Print and shaded views of the part. All mm, measured from the part's lowest x, y and z. A direction names the side the tool comes from. Round coordinates to 2 decimals unless told otherwise and drop trailing zeros. Loops run counter-clockwise (first coordinate to the right, second up) from the corner with the lowest first, then second, coordinate; pieces in that order, holes last. Notation, with made-up numbers: (22.25, 38.5) -> (56.25, 38.5) arc R28 ccw to (56.25, 71.5) -> close; hole circle Ø2 at (-31, -4). An arc over 180 degrees is marked (long way). Use a Markdown table: item, result.
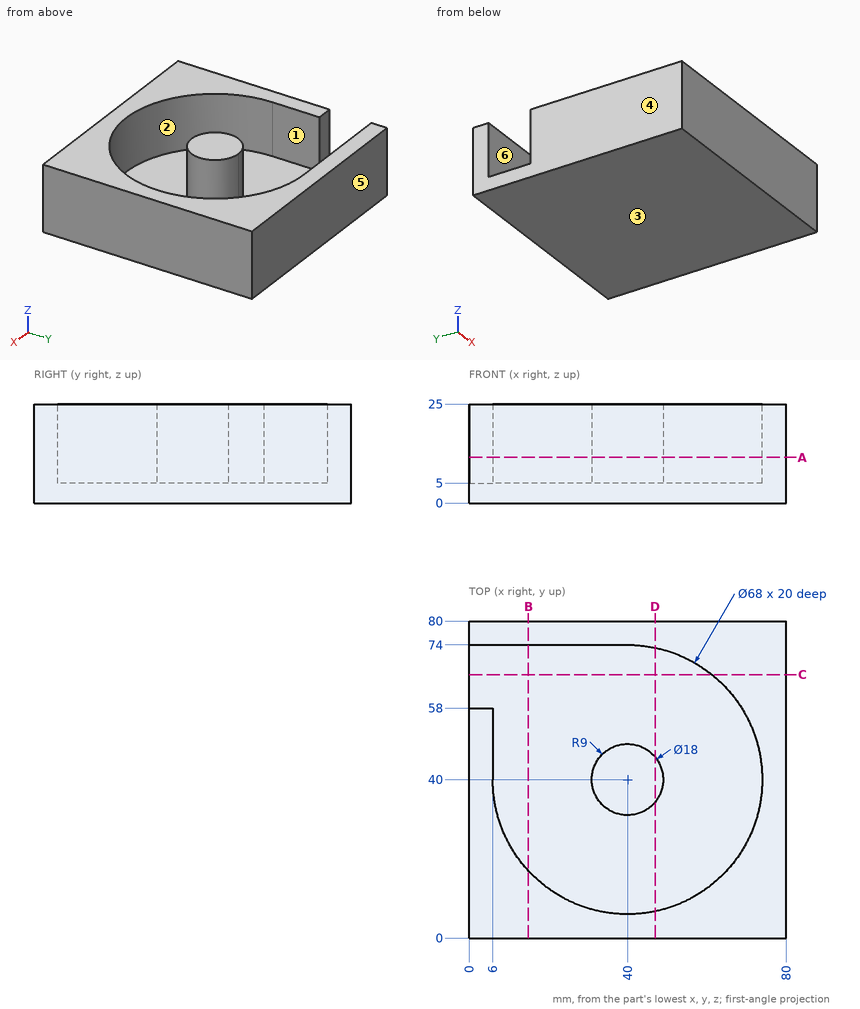
Q1. Drill centre lines: L1, parallel to Y at x = 40, z = 11; L2, parallel to Y at x = 9.5, z = 17. Where is each one in solid material? Low to high. Write a range as from..to.
Results list:
| item | result |
|---|---|
| L1 | y = 0..6, 31..49, 74..80 |
| L2 | y = 0..24.98, 74..80 |
Q2. Flat gauge pin, fed straight in: pin 1 (1.5 mm diameter, centred on x = 58, y = 52, fed in from +Z). Where does the tip first touch, or does it go through?
Results list:
| item | result |
|---|---|
| pin 1 | stops at z = 5 |
Q3. Band-saw the part on D-D, the plane x = 47. Give the cut face in (y, z), plus the area to 3 significant figures.
Results list:
| item | result |
|---|---|
| outline | (0, 0) -> (80, 0) -> (80, 25) -> (73.27, 25) -> (73.27, 5) -> (45.66, 5) -> (45.66, 25) -> (34.34, 25) -> (34.34, 5) -> (6.73, 5) -> (6.73, 25) -> (0, 25) -> close |
| area | 895 mm² |
Q4. Pull direction X, two halves, no side cores. Call the marked faces 1, 2, 3 and 4: released by +X, released by -X, zero draft, split by the parting line, or undercut.
Results list:
| item | result |
|---|---|
| face 1 | undercut |
| face 2 | undercut |
| face 3 | zero draft |
| face 4 | released by -X |
Q5. Band-saw the part on A-A, the plane z = 11.5. Give the cut face in (x, y), plus the area to 3 significant figures.
Results list:
| item | result |
|---|---|
| outline | (0, 0) -> (80, 0) -> (80, 80) -> (0, 80) -> (0, 74) -> (40, 74) arc R34 cw (long way) to (6, 40) -> (6, 58) -> (0, 58) -> close; circle Ø18 at (40, 40) |
| area | 2,680 mm² |
Q6. Tool access for the marked faces 5 and 6: list every direction of +Z, -Z, +X, -X, +Y, -Y with a clear straight run to the whole face (end or side of a thin tool).
Results list:
| item | result |
|---|---|
| face 5 | +Z, -Z, +X, -X, +Y |
| face 6 | +Z, -X |
Q7. Band-saw the part on B-B, the plane x = 15. Give the cut face in (y, z), plus the area to 3 significant figures.
Results list:
| item | result |
|---|---|
| outline | (0, 0) -> (80, 0) -> (80, 25) -> (74, 25) -> (74, 5) -> (16.96, 5) -> (16.96, 25) -> (0, 25) -> close |
| area | 859 mm² |
Q8. Band-saw the part on C-C, the plane y = 66.5. Give the cut face in (x, z).
Results list:
| item | result |
|---|---|
| outline | (0, 0) -> (80, 0) -> (80, 25) -> (61.3, 25) -> (61.3, 5) -> (0, 5) -> close |
